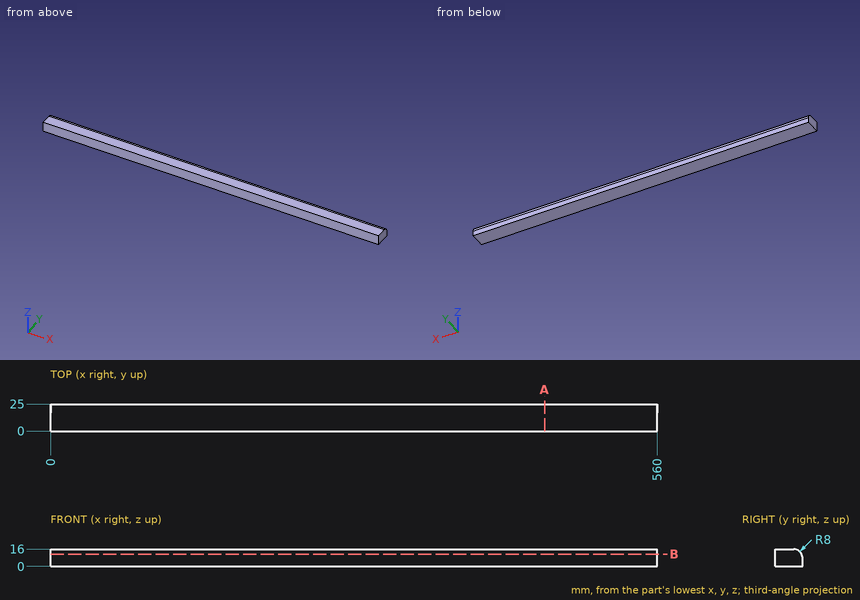
Verification items for this drawing (mm, ordinates from the low corner). Give positions to 0.01 mm unless a question says otherwise; leave off trailing zeros. Write each loop counter-clockwise with the first axis right and the second up, starting at its lowest first coordinate (ties: lowest second). Pieces come first, ordered by that corner, then holes.
1) Cross-section at A-A (x = 456). Record the boundary of the cut face in (y, z).
Values follow:
outline: (0, 0) - (25, 0) - (25, 8) arc R8 ccw to (17, 16) - (0, 16) - close
2) Cross-section at B-B (z = 11.25). Record the boundary of the cut face in (x, y).
Values follow:
outline: (0, 0) - (560, 0) - (560, 24.31) - (0, 24.31) - close
3) Thickness scan on line 1 (Y direction, x = 118.5, z = 9); line 2 (Z direction, x = 330.5, y = 17.5); line 3 (Y direction, x = 181, z = 13) (3 decimals). Record the ranges inside material, lowest first.
Values follow:
line 1: y = 0 to 24.94
line 2: z = 0 to 15.98
line 3: y = 0 to 23.245
